Drawing for the job (mm, zero at the part's lowest x, y, z). Coordinates: 2 decimals unless noted, no trailing zeros. Write each loop counter-clockwise with the first axis right and the second up, starting at its lowest first coordinate (ties: lowest second). Pieces come first, ordered by that corner, then holes. Notation, with made-up numbers: (15.5, 80) -> (72.5, 80) arc R26 cw to (72.5, 113) -> close; hole circle Ø8 at (-11.75, 29). An arc over 180 degrees is marked (long way). Write each question's results on one line, items separated by ' | '. Start each with the question number.
Q1. Drill centre lines: line 1 (X direction, y = 1.75, z = 50); line 2 (X direction, y = 3.1, z = 50); line 3 (X direction, y = 6.5, z = 46.5). Where is each one in solid material? Low to high.
Q2. Saw through at B-B on z = 20. Give the cut face in (x, y), and give its area (3 significant figures).
Q3. Drop flat-ended pins along their axis: pin 1 Ø3 at (y, z) = (2, 14) entering from +X; pin 2 Ø1.5 at (x, y) = (66.5, 2) entering from -Z; pin 3 Ø7 at (x, z) = (50, 50) entering from +Y; pin 4 Ø1.2 at (x, z) = (50, 34) entering from -Y. Give the stop position or say it passes through.
Q4. Two-plate mould, pull along X, no slides. Class the marked faces 1, 2 and 3: released by +X, released by -X, zero draft, split by the parting line, or undercut.
Q5. Saw through at A-A on x = 15. Give the cut face in (y, z).
Q6. Saw through at C-C on x = 90. Give the cut face in (y, z).
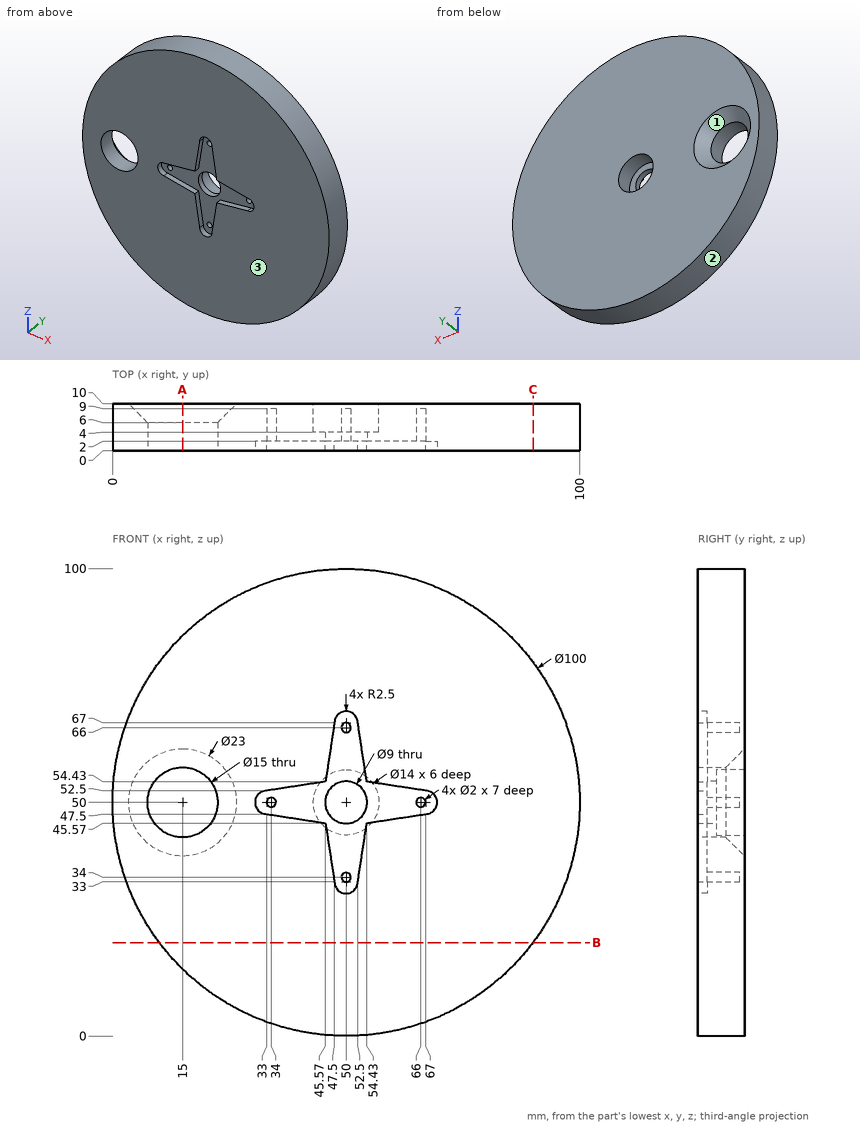
Returned:
1) line 1: x = 0 to 7.5, 22.5 to 30.5, 69.5 to 100 | line 2: x = 0 to 7.5, 22.5 to 33, 35 to 45.5, 54.5 to 65, 67 to 100 | line 3: x = 0.12 to 7.81, 22.19 to 43.94, 56.06 to 99.88
2) outline: (10, 0) -> (90, 0) -> (90, 10) -> (10, 10) -> close | area: 800 mm2
3) pin 1: stops at x = 86.19 | pin 2: stops at z = 2.55 | pin 3: passes through | pin 4: stops at y = 9
4) face 1: undercut | face 2: split by the parting line | face 3: zero draft
5) outline: (0, 14.29) -> (10, 14.29) -> (10, 38.5) -> (6, 42.5) -> (0, 42.5) -> close; (0, 57.5) -> (6, 57.5) -> (10, 61.5) -> (10, 85.71) -> (0, 85.71) -> close
6) outline: (0, 20) -> (10, 20) -> (10, 80) -> (0, 80) -> close
